Here's how the part is built. I have some questions about the finished solid (model axes, mm). Give positions to 0.01 mm unless a question says otherwise; leave off trailing zeros. Write each loop counter-clockwise with the first axis right and the second up, starting at its lowest first coordinate (ties: lowest second). Pieces come first, ordered by that corner, then holes. Notation, with made-up numbers: M 68.5,80.5 L 95.5,80.5 A27 cw 95.5,102.5 Z; hole C 24.5,47 d4. An arc over 180 degrees is marked long. Answer as CSV lines item,"result". Start each with the question number.
Q1. Suppose I cut it at A-A (y = 10.5). Write out the boundary of the cut face in (x, z), then the cut area to 3 significant figures.
Q2. Suppose I cut it at B-B (z = 0.75). Write out the boundary of the cut face in (x, y), then the cut area to 3 significant figures.
Q3. If I drill on line 1 along X through (y, z) = (9.25, 0.25); line 2 along X through (y, z) = (15, 1.1); line 3 along Y through (x, z) = (-3, 2.8), over which ranges is the centre line in solid material (lowest first)?
Q4. For pin 1 (8 mm diameter, centred on x = -55.5, y = 8, fed in from -Z); pin 2 (1.5 mm diameter, centred on x = 5, z = 1.5, fed in from -Y), each with a flat end and sliding along its axis, tell me the tip position at first contact or that it passes through.
```python
from build123d import *

# Parameters (mm, degrees)
P_IDAT_VYSUNUT_M1_DEPTH = 3


with BuildPart() as part:
    # Skica1 → Přidat vysunutím1 (new body)
    with BuildSketch(Plane.XY):
        with BuildLine():
            Line((-116.5, 0), (-13.5, 0))
            Line((-13.5, 0), (-13.5, 3))
            Line((-13.5, 3), (13.5, 3))
            Line((13.5, 3), (13.5, 0))
            Line((13.5, 0), (116.5, 0))
            Line((116.5, 0), (116.5, 16))
            Line((116.5, 16), (53.5, 16))
            Line((53.5, 16), (11.961316817, 16))
            ThreePointArc((11.961316817, 16), (0, 7.13), (-11.961316817, 16))
            Line((-11.961316817, 16), (-53.5, 16))
            Line((-53.5, 16), (-116.5, 16))
            Line((-116.5, 16), (-116.5, 0))
        make_face()
    extrude(amount=P_IDAT_VYSUNUT_M1_DEPTH)


solid = part.part
```
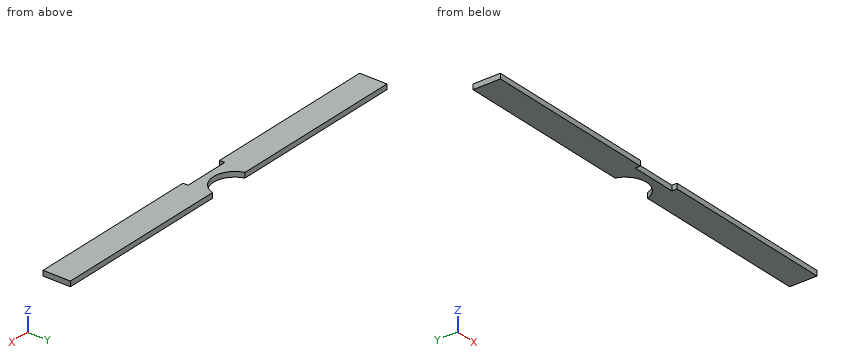
Resolved:
1,outline,"M -116.5,0 L -8.54,0 L -8.54,3 L -116.5,3 Z; M 8.54,0 L 116.5,0 L 116.5,3 L 8.54,3 Z"
1,area,"648 mm^2"
2,outline,"M -116.5,0 L -13.5,0 L -13.5,3 L 13.5,3 L 13.5,0 L 116.5,0 L 116.5,16 L 11.96,16 A12.5 cw -11.96,16 L -116.5,16 Z"
2,area,"3,490 mm^2"
3,line 1,"-116.5 to -6.96, 6.96 to 116.5"
3,line 2,"-116.5 to -11.61, 11.61 to 116.5"
3,line 3,"3 to 7.5"
4,pin 1,"z = 0"
4,pin 2,"y = 3"
